Could you check a few things on this model? Use its own coordinates, in mm. A direction names the side the tool comes from. Round coordinates to 2 decimals unless told otherwise and drop trailing zeros. Loops run counter-clockwise (first coordinate to the right, second up) from the corner with the lowest first, then second, coordinate; pieces in that order, holes last. Notation, with made-up numbers: M 64,-30.75 L 110,-30.75 A33 ccw 110,-1.75 Z; hole C -22.5,24 d7. An arc over 180 degrees is marked long. One line per item, written item: value. Start each with the question number.
Q1. I'm going to push flat-ended pins straight in: pin 1 Ø0.8 at (x, y) = (-2.5, -5) entering from +Z; pin 2 Ø12 at (y, z) = (-1, 223) entering from +X; pin 3 Ø4 at (y, z) = (6.5, 125.5) entering from -X; pin 4 Ø1.5 at (y, z) = (8, 109) entering from +X. Where does each tip first touch, or does it pass through?
Q2. Please list where these lines run through material, in increasing order: line 1 along Z through (x, y) = (11.5, 1.5); line 2 along Z through (x, y) = (3.25, 5); line 3 along Y through (x, z) = (0, 196).
Q3. Which directions (+Z, -Z, +X, -X, +Y, -Y) give clear straight access to the entire face, cutting with the end or side of a thin tool? Please do faces 1 (the face through (4.72, 1.49, 380.92)), 2 (the face through (-0.1, -5.2, 371.8)).
Q4. Imagine slicing it at A-A (z = 57.5). Please give me the cut outline in (x, y), then the cut area to 3 significant figures.
from build123d import *

# Parameters (mm, degrees)
SKETCH1_R           = 12.5
PISTON_DEPTH        = 5
SKETCH2_R           = 6
ROD_DEPTH           = 389
THREADS_START       = -18
SKETCH3_R           = 6
SKETCH3_R_2         = 5
THREADS_DEPTH       = 18
ROD_CHAMFER_SIZE    = 1
WRENCH_FLAT_DEPTH   = 390.401463788
THREAD_CHAMFER_SIZE = 0.5
CUT_EXTRUDE1_START  = -15.5
SKETCH5_R           = 5
SKETCH5_R_2         = 4.95
CUT_EXTRUDE1_DEPTH  = 15.5


with BuildPart() as part:
    # Sketch1 → Piston (new body)
    with BuildSketch(Plane.XY):
        Circle(SKETCH1_R)
    extrude(amount=PISTON_DEPTH)

    # Sketch2 → Rod (add)
    with BuildSketch(Plane.XY):
        Circle(SKETCH2_R)
    extrude(amount=ROD_DEPTH)

    # Sketch3 → Threads (cut)
    with BuildSketch(Plane.XY.offset(389).offset(THREADS_START)):
        Circle(SKETCH3_R)
        Circle(SKETCH3_R_2, mode=Mode.SUBTRACT)
    extrude(amount=THREADS_DEPTH, mode=Mode.SUBTRACT)

    # Rod Chamfer
    rod_chamfer_edges = [part.edges().sort_by_distance(p)[0] for p in [
        (-5, 0, 371),
    ]]
    chamfer(rod_chamfer_edges, length=ROD_CHAMFER_SIZE - 0.0001)  # a hair under: the kernel refuses the full size

    # Sketch4 → Wrench Flat (cut, symmetric)
    with BuildSketch(Plane(origin=(0, 0, 0), x_dir=(1, 0, 0), z_dir=(0, 1, 0))):
        Polygon((5, -372), (5, -367), (6, -366), (6, -372), align=None)
    wrench_flat = extrude(amount=WRENCH_FLAT_DEPTH, both=True, mode=Mode.SUBTRACT)

    # Mirror1: Wrench Flat across plane
    add(wrench_flat.mirror(Plane(origin=(0, 0, 0), x_dir=(0, 0, 1), z_dir=(1, 0, 0))), mode=Mode.SUBTRACT)

    # Thread Chamfer
    thread_chamfer_edges = [part.edges().sort_by_distance(p)[0] for p in [
        (-5, 0, 389),
    ]]
    chamfer(thread_chamfer_edges, length=THREAD_CHAMFER_SIZE)

    # Sketch5 → Cut-Extrude1 (cut)
    with BuildSketch(Plane.XY.offset(389).offset(CUT_EXTRUDE1_START)):
        Circle(SKETCH5_R)
        Circle(SKETCH5_R_2, mode=Mode.SUBTRACT)
    extrude(amount=CUT_EXTRUDE1_DEPTH, mode=Mode.SUBTRACT)


solid = part.part
Report:
1. pin 1: stops at z = 371.81
1. pin 2: stops at x = 6
1. pin 3: stops at x = -3.97
1. pin 4: passes through
2. line 1: z = 0 to 5
2. line 2: z = 0 to 371.04
2. line 3: y = -6 to 6
3. face 1: +Z
3. face 2: +Z, -Y
4. outline: C 0,0 d12
4. area: 113 mm²
